from build123d import *

# Parameters (mm, degrees)
SKETCH_1_R          = 10
EXTRUDE_1_DEPTH     = 2
SKETCH_2_R          = 4.5
EXTRUDE_2_DEPTH     = 2.5
SKETCH_3_R          = 1.5
CUT_EXTRUDE_1_DEPTH = 2.5
SKETCH_4_R          = 1.5
CUT_EXTRUDE_2_DEPTH = 15.84082208


with BuildPart() as part:
    # 草图1 → 凸台-拉伸1 (new body)
    with BuildSketch(Plane.XY):
        Circle(SKETCH_1_R)
    extrude(amount=EXTRUDE_1_DEPTH)

    # 草图2 → 凸台-拉伸2 (add)
    with BuildSketch(Plane.XY.offset(2)):
        Circle(SKETCH_2_R)
    extrude(amount=EXTRUDE_2_DEPTH)

    # 草图3 → 切除-拉伸1 (cut)
    with BuildSketch(Plane(origin=(0, 0, 0), x_dir=(-1, 0, 0), z_dir=(0, 0, -1))):
        with Locations((0, 7)):
            Circle(SKETCH_3_R)
        with Locations((7, 0)):
            Circle(SKETCH_3_R)
        with Locations((0, -7)):
            Circle(SKETCH_3_R)
        with Locations((-7, 0)):
            Circle(SKETCH_3_R)
    extrude(amount=-CUT_EXTRUDE_1_DEPTH, mode=Mode.SUBTRACT)

    # 草图4 → 切除-拉伸2 (cut, through all)
    with BuildSketch(Plane(origin=(0, 0, 0), x_dir=(-1, 0, 0), z_dir=(0, 0, -1))):
        Circle(SKETCH_4_R)
    extrude(amount=-CUT_EXTRUDE_2_DEPTH, mode=Mode.SUBTRACT)


solid = part.part
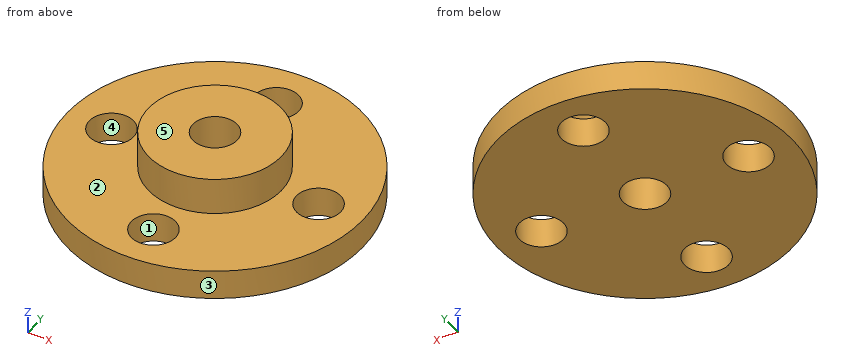
Verification items for the finished model (mm, model axes). Face numbers are marked on the shaded views. A direction names the side the tool comes from. Coordinates: 2 decimals unless noted, no trailing zeros. Order: outer loops, then holes, each group sorted by start corner. A loop starts at its lowest first (then second) coordinate and runs counter-clockwise, first axis right, second up.
Item 1: Depth check by flat-ended pin: pin 1 (4 mm diameter, centred on x = -6.5, y = 8, fed in from -Z); pin 2 (4 mm diameter, centred on x = -7, y = 0, fed in from +Z). Enter the tip coordinate at first touch or a pass-through.
Filled in:
pin 1: stops at z = 0
pin 2: stops at z = 2
Item 2: Material ranges on L1, parallel to Y at x = 0, z = 1.25; L2, parallel to X at y = -1, z = 0.3; L3, parallel to Z at x = -5, y = 5, recorded low to high.
Filled in:
L1: y = -10 to -8.5, -5.5 to -1.5, 1.5 to 5.5, 8.5 to 10
L2: x = -9.95 to -8.12, -5.88 to -1.12, 1.12 to 5.88, 8.12 to 9.95
L3: z = 0 to 2
Item 3: Section check B-B, the plane y = -0.5. Enter the section's corners in (x, z), then the cut area to 3 significant figures.
Filled in:
outline: (-9.99, 0) - (-8.41, 0) - (-8.41, 2) - (-9.99, 2) - close; (-5.59, 0) - (-1.41, 0) - (-1.41, 4.5) - (-4.47, 4.5) - (-4.47, 2) - (-5.59, 2) - close; (1.41, 0) - (5.59, 0) - (5.59, 2) - (4.47, 2) - (4.47, 4.5) - (1.41, 4.5) - close; (8.41, 0) - (9.99, 0) - (9.99, 2) - (8.41, 2) - close
area: 38.3 mm2
Item 4: Section check C-C, the plane y = -8. Enter the section's corners in (x, z), then the cut area to 3 significant figures.
Filled in:
outline: (-6, 0) - (-1.12, 0) - (-1.12, 2) - (-6, 2) - close; (1.12, 0) - (6, 0) - (6, 2) - (1.12, 2) - close
area: 19.5 mm2
Item 5: Section check A-A, the plane x = 0. Enter the section's corners in (y, z), then the cut area to 3 significant figures.
Filled in:
outline: (-10, 0) - (-8.5, 0) - (-8.5, 2) - (-10, 2) - close; (-5.5, 0) - (-1.5, 0) - (-1.5, 4.5) - (-4.5, 4.5) - (-4.5, 2) - (-5.5, 2) - close; (1.5, 0) - (5.5, 0) - (5.5, 2) - (4.5, 2) - (4.5, 4.5) - (1.5, 4.5) - close; (8.5, 0) - (10, 0) - (10, 2) - (8.5, 2) - close
area: 37.0 mm2
Item 6: Release check for a two-part mould opening along X. For the marked faces 3, 4 and 5 record: +X half, -X half, draft (parallel to the pull), parting line (faces both ways), or undercut.
Filled in:
face 3: parting line
face 4: undercut
face 5: draft
Item 7: Section check D-D, the plane z = 3.15. Enter the section's corners in (x, y), then the cut area to 3 significant figures.
Filled in:
outline: circle Ø9 at (0, 0); hole circle Ø3 at (0, 0)
area: 56.5 mm2
Item 8: Access from +Z, -Z, +X, -X, +Y, -Y to the whole of each face (thin tool, end or side, straight path). Record for the marked faces 1 and 2.
Filled in:
face 1: +Z, -Z
face 2: +Z
